Check sheet for the modelled part. Datum: model origin and axes. Units: mm. A direction names the side the tool comes from. Round coordinates to 2 decimals unless told otherwise and drop trailing zeros. Loops run counter-clockwise (first coordinate to the right, second up) from the corner with the lowest first, then second, coordinate; pieces in that order, holes last. Notation, with made-up numbers: (61, 42.5) -> (66, 42.5) arc R23 ccw to (66, 53.5) -> close; hole circle Ø6 at (34.5, -13.75). An arc over 180 degrees is marked (long way). Use one line per item in the form item = value. Start each with the question number.
(1) Sectioned sample at A-A (y = 0). Record the cut outline in (x, z).
(2) Sectioned sample at D-D (y = -35). Record the cut outline in (x, z), and give its area (3 significant figures).
(3) Set-up check for faces 4 (the flat face through (40, 0, 20)), 5 (the flat face through (20, 13, 20)), 6 (the flat face through (19, -11, 20)): record each of +Z, -Z, +X, -X, +Y, -Y from which the full face is reachable in a straight line by a thin tool's end or side.
(4) Sectioned sample at C-C (x = 35). Record the cut outline in (y, z), and give its area (3 significant figures).
(5) Material ranges on probe 1 along Y at (x, z) = (39.1, 30); probe 2 along Y at (x, z) = (19.5, 11); probe 3 along Y at (x, z) = (-5, 1.5), recorded low to high. Write a range as [from, to].
(6) Draft check along X on faces 1 (the cylindrical face through (-47.954, 2.11, 1.479)), 2 (the cylindrical face through (-3, 0, 2)), 3 (the flat face through (38, 0, 20)). Enter one of: released by +X, released by -X, zero draft, split by the parting line, or undercut.
(7) Go/stop test with flat-tipped pins: pin 1 (7 mm diameter, centred on y = 0, z = 25, fed in from -X); pin 2 (6.5 mm diameter, centred on x = -35, y = 0, fed in from +Z); pin 3 (3 mm diameter, centred on x = 22.5, z = 29.5, fed in from -Y). Record where each tip stops, or that it passes through.
(8) Sectioned sample at B-B (z = 25). Record the cut outline in (x, y), and give its area (3 significant figures).
from build123d import *

# Parameters (mm, degrees)
SKETCH_3_R          = 48
EXTRUDE_2_DEPTH     = 3
SKETCH_4_R          = 3
CUT_EXTRUDE_1_DEPTH = 3
EXTRUDE_3_DEPTH     = 35
SKETCH_6_R          = 3
SKETCH_6_R_2        = 1.5
CUT_EXTRUDE_2_DEPTH = 35
SKETCH_7_R          = 1.55
CUT_EXTRUDE_5_DEPTH = 35
SKETCH_8_R          = 2.05
CUT_EXTRUDE_6_DEPTH = 10
SKETCH_9_R          = 1.55
CUT_EXTRUDE_7_DEPTH = 10


with BuildPart() as part:
    # 草图3 → 凸台-拉伸2 (new body)
    with BuildSketch(Plane.XY):
        Circle(SKETCH_3_R)
    extrude(amount=EXTRUDE_2_DEPTH)

    # 草图4 → 切除-拉伸1 (cut)
    with BuildSketch(Plane.XY.offset(3)):
        Circle(SKETCH_4_R)
    extrude(amount=-CUT_EXTRUDE_1_DEPTH, mode=Mode.SUBTRACT)

    # 草图5 → 凸台-拉伸3 (add)
    with BuildSketch(Plane.XY.offset(3)):
        with BuildLine():
            ThreePointArc((0, 12.5), (0.146446609, 12.853553391), (0.5, 13))
            Line((0.5, 13), (39.5, 13))
            ThreePointArc((39.5, 13), (39.853553391, 12.853553391), (40, 12.5))
            Line((40, 12.5), (40, -12.5))
            ThreePointArc((40, -12.5), (39.853553391, -12.853553391), (39.5, -13))
            Line((39.5, -13), (0.5, -13))
            ThreePointArc((0.5, -13), (0.146446609, -12.853553391), (0, -12.5))
            Line((0, -12.5), (0, -11.5))
            ThreePointArc((0, -11.5), (0.146446609, -11.146446609), (0.5, -11))
            Line((0.5, -11), (37.5, -11))
            ThreePointArc((37.5, -11), (37.853553391, -10.853553391), (38, -10.5))
            Line((38, -10.5), (38, 0))
            Line((38, 0), (38, 10.5))
            ThreePointArc((38, 10.5), (37.853553391, 10.853553391), (37.5, 11))
            Line((37.5, 11), (0.5, 11))
            ThreePointArc((0.5, 11), (0.146446609, 11.146446609), (0, 11.5))
            Line((0, 11.5), (0, 12.5))
        make_face()
    extrude(amount=EXTRUDE_3_DEPTH)

    # 草图6 → 切除-拉伸2 (cut)
    with BuildSketch(Plane(origin=(40, 0, 0), x_dir=(0, 0, -1), z_dir=(1, 0, 0))):
        with Locations((-25, 0)):
            Circle(SKETCH_6_R)
        with Locations((-20, -5)):
            Circle(SKETCH_6_R_2)
        with Locations((-20, 5)):
            Circle(SKETCH_6_R_2)
        with Locations((-30, -5)):
            Circle(SKETCH_6_R_2)
        with Locations((-30, 5)):
            Circle(SKETCH_6_R_2)
    extrude(amount=-CUT_EXTRUDE_2_DEPTH, mode=Mode.SUBTRACT)

    # 草图7 → 切除-拉伸5 (cut)
    with BuildSketch(Plane.XY.offset(3)):
        with Locations((-35, 0)):
            Circle(SKETCH_7_R)
        with Locations((-24.748737342, 24.748737342)):
            Circle(SKETCH_7_R)
        with Locations((0, 35)):
            Circle(SKETCH_7_R)
        with Locations((24.748737342, 24.748737342)):
            Circle(SKETCH_7_R)
        with Locations((35, 0)):
            Circle(SKETCH_7_R)
        with Locations((24.748737342, -24.748737342)):
            Circle(SKETCH_7_R)
        with Locations((0, -35)):
            Circle(SKETCH_7_R)
        with Locations((-24.748737342, -24.748737342)):
            Circle(SKETCH_7_R)
    extrude(amount=-CUT_EXTRUDE_5_DEPTH, mode=Mode.SUBTRACT)

    # 草图8 → 切除-拉伸6 (cut)
    with BuildSketch(Plane.XY.offset(3)):
        with Locations((0, 35)):
            Circle(SKETCH_8_R)
        with Locations((24.748737342, 24.748737342)):
            Circle(SKETCH_8_R)
        with Locations((35, 0)):
            Circle(SKETCH_8_R)
        with Locations((24.748737342, -24.748737342)):
            Circle(SKETCH_8_R)
        with Locations((0, -35)):
            Circle(SKETCH_8_R)
        with Locations((-24.748737342, -24.748737342)):
            Circle(SKETCH_8_R)
        with Locations((-35, 0)):
            Circle(SKETCH_8_R)
        with Locations((-24.748737342, 24.748737342)):
            Circle(SKETCH_8_R)
    extrude(amount=-CUT_EXTRUDE_6_DEPTH, mode=Mode.SUBTRACT)

    # 草图9 → 切除-拉伸7 (cut)
    with BuildSketch(Plane.XY.offset(3)):
        with Locations((-5, 5)):
            Circle(SKETCH_9_R)
        with Locations((5, 5)):
            Circle(SKETCH_9_R)
        with Locations((5, -5)):
            Circle(SKETCH_9_R)
        with Locations((-5, -5)):
            Circle(SKETCH_9_R)
    extrude(amount=-CUT_EXTRUDE_7_DEPTH, mode=Mode.SUBTRACT)


solid = part.part
Checks:
q1.outline = (-48, 0) -> (-37.05, 0) -> (-37.05, 3) -> (-48, 3) -> close; (-32.95, 0) -> (-3, 0) -> (-3, 3) -> (-32.95, 3) -> close; (3, 0) -> (32.95, 0) -> (32.95, 3) -> (3, 3) -> close; (37.05, 0) -> (48, 0) -> (48, 3) -> (40, 3) -> (40, 22) -> (38, 22) -> (38, 3) -> (37.05, 3) -> close; (38, 28) -> (40, 28) -> (40, 38) -> (38, 38) -> close
q2.outline = (-32.85, 0) -> (-2.05, 0) -> (-2.05, 3) -> (-32.85, 3) -> close; (2.05, 0) -> (32.85, 0) -> (32.85, 3) -> (2.05, 3) -> close
q2.area = 185 mm2
q3.face_4 = +Z, +X, +Y, -Y
q3.face_5 = +Z, +X, -X, +Y
q3.face_6 = +Z, -X
q4.outline = (-32.85, 0) -> (-2.05, 0) -> (-2.05, 3) -> (-11, 3) -> (-11, 38) -> (-13, 38) -> (-13, 3) -> (-32.85, 3) -> close; (2.05, 0) -> (32.85, 0) -> (32.85, 3) -> (13, 3) -> (13, 38) -> (11, 38) -> (11, 3) -> (2.05, 3) -> close
q4.area = 325 mm2
q5.probe_1 = [-13, -6.5], [-3.5, 3.5], [6.5, 13]
q5.probe_2 = [-13, -11], [11, 13]
q5.probe_3 = [-47.74, -6.55], [-3.45, 3.45], [6.55, 47.74]
q6.face_1 = split by the parting line
q6.face_2 = undercut
q6.face_3 = released by -X
q7.pin_1 = 38
q7.pin_2 = 3
q7.pin_3 = -13
q8.outline = (0, -12.5) arc R0.5 ccw to (0.5, -13) -> (39.5, -13) arc R0.5 ccw to (40, -12.5) -> (40, -3) -> (38, -3) -> (38, -10.5) arc R0.5 cw to (37.5, -11) -> (0.5, -11) arc R0.5 ccw to (0, -11.5) -> close; (0, 11.5) arc R0.5 ccw to (0.5, 11) -> (37.5, 11) arc R0.5 cw to (38, 10.5) -> (38, 3) -> (40, 3) -> (40, 12.5) arc R0.5 ccw to (39.5, 13) -> (0.5, 13) arc R0.5 ccw to (0, 12.5) -> close
q8.area = 192 mm2
